from build123d import *

# Parameters (mm, degrees)
F1_DEPTH = 25.4
F3_D     = 6.35


with BuildPart() as f1:
    # F0 (on Front) → F1 (new body)
    with BuildSketch(Plane.XZ):
        with BuildLine():
            Line((-12.7, 75.068495), (-25.022832, 4.360951))
            ThreePointArc((-25.022832, 4.360951), (-2.188615, -25.305532), (25.4, 0))
            ThreePointArc((25.4, 0), (25.305532, 2.188615), (25.022832, 4.360951))
            Line((25.022832, 4.360951), (12.7, 75.068495))
            Line((12.7, 75.068495), (-12.7, 75.068495))
        make_face()
    extrude(amount=-F1_DEPTH)

    # F3 (through all)
    with Locations(Plane.XZ):
        with Locations((0, -12.7), (0, 62.368495)):
            Hole(F3_D / 2)


solid = f1.part
Could you check a few things on this model? Use its own coordinates, in mm. Give positions to 0.01 mm unless a question says otherwise; leave off trailing zeros. Order: outer loops, then holes, each group sorted by start corner. A loop starts at its lowest first (then second) coordinate and runs counter-clockwise, first axis right, second up. Notation, with made-up numbers: M 16,56.5 L 62,56.5 A25 cw 62,84.5 Z; hole C 76.25,2.25 d7. An arc over 180 degrees is marked long. One line per question, with ' | ' between items.
1. I want a section at C-C (y = 15.5). Give the number of separate pieces and of enclosed holes in the cut face, and give its area (3 significant figures).
Results:
separate pieces: 1 | enclosed holes: 2 | area: 3,840 mm²
2. We'd pull the mould along X, two halves only. Please class faces 1 (the face through (25.308, 12.522, 2.158)), 2 (the face through (0.69, 12.88, 59.27)), 3 (the face through (0, 13, 75.068)): +X half, -X half, draft (parallel to the pull), parting line (faces both ways), or undercut.
Results:
face 1: +X half | face 2: undercut | face 3: draft
3. If I drill on line 1 (Z direction, x = 0, y = 7.25) (1 decimal); line 2 (Z direction, x = -2, y = 17.5); line 3 (X direction, y = 11.5, z = 63.5), over which ranges is the centre line in solid material (lowest first)?
Results:
line 1: -25.4 to -15.9, -9.5 to 59.2, 65.5 to 75.1 | line 2: -25.32 to -15.17, -10.23 to 59.9, 64.83 to 75.07 | line 3: -14.72 to -2.97, 2.97 to 14.72
4. I'm going to push flat-ended pins straight in: pin 1 (4 mm diameter, centred on x = -17.5, z = -4, fed in from -Y); pin 2 (4 mm diameter, centred on y = 11.5, z = 26, fed in from +X); pin 3 (4 mm diameter, centred on x = 0, z = 62.37, fed in from -Y); pin 4 (6 mm diameter, centred on y = 4.5, z = 46, fed in from -X). Where does each tip first touch, or does it pass through?
Results:
pin 1: y = 0 | pin 2: x = 21.6 | pin 3: through | pin 4: x = -18.29
5. I want a section at D-D (z = 48.5). List the corners of the cut face in (x, y) for me.
Results:
outline: M -17.33,0 L 17.33,0 L 17.33,25.4 L -17.33,25.4 Z
6. I want a section at A-A (x = 0). List the corners of the cut face in (y, z) for me (1 decimal).
Results:
outline: M 0,-25.4 L 25.4,-25.4 L 25.4,-15.9 L 0,-15.9 Z; M 0,-9.5 L 25.4,-9.5 L 25.4,59.2 L 0,59.2 Z; M 0,65.5 L 25.4,65.5 L 25.4,75.1 L 0,75.1 Z
7. I want a section at B-B (z = -12.7). List the corners of the cut face in (x, y) for me (3 decimals).
Results:
outline: M -21.997,0 L -3.175,0 L -3.175,25.4 L -21.997,25.4 Z; M 3.175,0 L 21.997,0 L 21.997,25.4 L 3.175,25.4 Z
